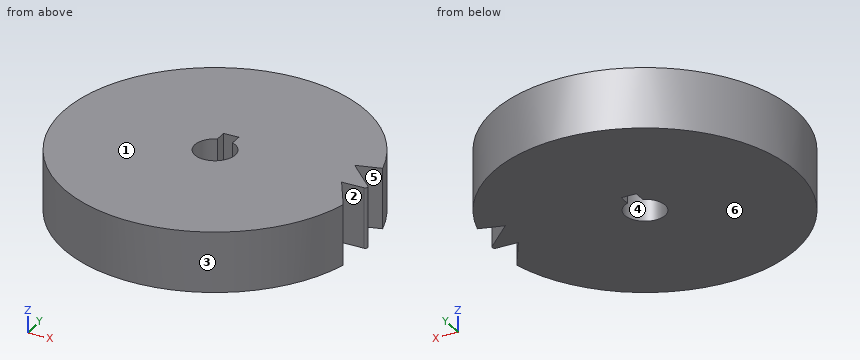
from build123d import *

# Parameters (mm, degrees)
SKETCH1_R          = 30
EXTRUDE1_DEPTH     = 12
CUT_EXTRUDE1_DEPTH = 12


with BuildPart() as part:
    # Sketch1 → Extrude1 (new body)
    with BuildSketch(Plane.XY):
        Circle(SKETCH1_R)
        with BuildLine():
            Line((-1.5, 6), (1.5, 6))
            Line((1.5, 6), (1.5, 3.708099244))
            ThreePointArc((1.5, 3.708099244), (0, -4), (-1.5, 3.708099244))
            Line((-1.5, 3.708099244), (-1.5, 6))
        make_face(mode=Mode.SUBTRACT)
    extrude(amount=EXTRUDE1_DEPTH)

    # Sketch2 → Cut-Extrude1 (cut)
    with BuildSketch(Plane.XY.offset(12)):
        with BuildLine():
            Line((25, 0), (29.411515004, 0))
            ThreePointArc((29.411515004, 0), (29.87345477, 0.308658284), (29.765068394, 0.853553391))
            Line((29.765068394, 0.853553391), (24.148145657, 6.470476128))
            Line((24.148145657, 6.470476128), (34.591694707, 9.268816662))
            Line((34.591694707, 9.268816662), (29.575317547, -7.924682453))
            Line((29.575317547, -7.924682453), (25, 0))
        make_face()
    extrude(amount=-CUT_EXTRUDE1_DEPTH, mode=Mode.SUBTRACT)


solid = part.part
Model file for the job. Use its own axes, mm. Face numbers are marked on the shaded views. A direction names the side the tool comes from. Round coordinates to 2 decimals unless told otherwise and drop trailing zeros. Order: outer loops, then holes, each group sorted by start corner. A loop starts at its lowest first (then second) coordinate and runs counter-clockwise, first axis right, second up.
(1) Band-saw the part on B-B (z = 3). List the corners of the cut face in (x, y).
(2) Pull direction X, two halves, no side cores. Call the marked faces 3, 4, 5 and 6: released by +X, released by -X, zero draft, split by the parting line, or undercut.
(3) Pin check, flat tips, straight feed: pin 1 (5 mm diameter, centred on y = -22.5, z = 6, fed in from +X); pin 2 (5 mm diameter, centred on y = 15.5, z = 4, fed in from -X); pin 3 (4 mm diameter, centred on x = -16.5, z = 4.5, fed in from +Y); pin 4 (9 mm diameter, centred on x = 0, y = 0, fed in from -Z). Stop position of each tip, or through.
(4) Band-saw the part on A-A (x = 0). List the corners of the cut face in (y, z), then the cut area to 3 significant figures.
(5) Drill centre lines: line 1 (Y direction, x = 0, z = 6.25); line 2 (X direction, y = 4.5, z = 8.5); line 3 (Y direction, x = 21.5, z = 6.75). Where is each one in solid material? Low to high.
(6) Band-saw the part on D-D (y = -5.5). List the corners of the cut face in (x, z), then the cut area to 3 significant figures.
(7) 3-axis set-ups, long thin cutter, end or side, ignore diameter. For the marked faces 1 and 2: which of +Z, -Z, +X, -X, +Y, -Y reach the whole face in a straight line?
(8) Band-saw the part on C-C (x = 26.5). List the corners of the cut face in (y, z).
Verdict:
1. outline: (24.15, 6.47) - (28.98, 7.76) arc R30 ccw (long way) to (29.13, -7.16) - (25, 0) - (29.41, 0) arc R0.5 ccw to (29.77, 0.85) - close; hole (-1.5, 3.71) arc R4 ccw (long way) to (1.5, 3.71) - (1.5, 6) - (-1.5, 6) - close
2. face 3: split by the parting line
2. face 4: undercut
2. face 5: released by +X
2. face 6: zero draft
3. pin 1: stops at x = 22.36
3. pin 2: stops at x = -27.04
3. pin 3: stops at y = 26.26
3. pin 4: stops at z = 0
4. outline: (-30, 0) - (-4, 0) - (-4, 12) - (-30, 12) - close; (6, 0) - (30, 0) - (30, 12) - (6, 12) - close
4. area: 600 mm2
5. line 1: y = -30 to -4, 6 to 30
5. line 2: x = -29.66 to -1.5, 1.5 to 26.12
5. line 3: y = -20.92 to 20.92
6. outline: (-29.49, 0) - (28.18, 0) - (28.18, 12) - (-29.49, 12) - close
6. area: 692 mm2
7. face 1: +Z, +X, -X, +Y, -Y
7. face 2: +Z, -Z, +X
8. outline: (-14.06, 0) - (-2.6, 0) - (-2.6, 12) - (-14.06, 12) - close; (0, 0) - (4.12, 0) - (4.12, 12) - (0, 12) - close; (7.1, 0) - (14.06, 0) - (14.06, 12) - (7.1, 12) - close
